```python
from build123d import *

# Parameters (mm, degrees)
SKETCH1_W                   = 76.2
SKETCH1_H                   = 86.36
BOSS_EXTRUDE1_DEPTH         = 12.7
FILLET1_R                   = 3.81
CHAMFER1_SIZE               = 1.27
CUT_EXTRUDE1_DEPTH          = 10.16
SKETCH5_W                   = 16.51
SKETCH5_H                   = 11.43
CUT_EXTRUDE2_DEPTH          = 2.54
CUT_EXTRUDE3_REACH          = 117.87
SKETCH6_W                   = 16.51
SKETCH6_H                   = 7.62
CUT_EXTRUDE4_REACH          = 117.87
SKETCH8_W                   = 8.128
SKETCH8_H                   = 1.27
CUT_EXTRUDE5_REACH          = 117.87
SKETCH9_W                   = 10.16
SKETCH9_H                   = 3.81
CUT_EXTRUDE6_REACH          = 117.87
SKETCH10_W                  = 10.16
SKETCH10_H                  = 7.62
CUT_EXTRUDE7_REACH          = 117.87
SKETCH11_W                  = 26.67
SKETCH11_H                  = 15.24
F_1_4_20_TAPPED_HOLE1_D     = 5.1054
F_1_4_20_TAPPED_HOLE1_DEPTH = 6.35
F_1_4_20_TAPPED_HOLE1_TIP   = 1.533816902


with BuildPart() as part:
    # Sketch1 → Boss-Extrude1 (new body)
    with BuildSketch(Plane(origin=(0, 0, 0), x_dir=(1, 0, 0), z_dir=(0, 1, 0))):
        with Locations((38.1, 43.18)):
            Rectangle(SKETCH1_W, SKETCH1_H)
    extrude(amount=BOSS_EXTRUDE1_DEPTH)

    # Fillet1
    fillet1_edges = [part.edges().sort_by_distance(p)[0] for p in [
        (0, 6.35, -86.36),
        (76.2, 6.35, -86.36),
        (76.2, 6.35, 0),
        (0, 6.35, 0),
    ]]
    fillet(fillet1_edges, radius=FILLET1_R)

    # Chamfer1
    chamfer1_edges = [part.edges().sort_by_distance(p)[0] for p in [
        (0, 12.7, -43.18),
        (38.1, 12.7, -86.36),
        (38.1, 12.7, 0),
        (76.2, 12.7, -43.18),
        (1.115923164, 12.7, -1.115923164),
        (75.084076836, 12.7, -1.115923164),
        (75.084076836, 12.7, -85.244076836),
        (1.115923164, 12.7, -85.244076836),
    ]]
    chamfer(chamfer1_edges, length=CHAMFER1_SIZE)

    # Sketch4 → Cut-Extrude1 (cut)
    with BuildSketch(Plane.XZ):
        Polygon((3.81, -16.51), (16.51, -16.51), (16.51, -3.81), (59.69, -3.81), (59.69, -16.51), (72.39, -16.51), (72.39, -69.85), (59.69, -69.85), (59.69, -82.55), (16.51, -82.55), (16.51, -69.85), (3.81, -69.85), align=None)
    extrude(amount=-CUT_EXTRUDE1_DEPTH, mode=Mode.SUBTRACT)

    # Sketch5 → Cut-Extrude2 (cut)
    with BuildSketch(Plane(origin=(0, 12.7, 0), x_dir=(1, 0, 0), z_dir=(0, 1, 0))):
        with Locations((38.1, 10.795)):
            Rectangle(SKETCH5_W, SKETCH5_H)
    extrude(amount=-CUT_EXTRUDE2_DEPTH, mode=Mode.SUBTRACT)

    # Sketch6 → Cut-Extrude3 (cut, up to next)
    with BuildSketch(Plane.XY, mode=Mode.PRIVATE) as cut_extrude3_sk1:
        with Locations((38.1, 3.81)):
            Rectangle(SKETCH6_W, SKETCH6_H)
    cut_extrude3_tool1 = extrude(cut_extrude3_sk1.sketch, amount=-CUT_EXTRUDE3_REACH, mode=Mode.PRIVATE) & part.part
    add(cut_extrude3_tool1.solids().sort_by_distance((38.1, 3.81, 0))[0], mode=Mode.SUBTRACT)

    # Sketch8 → Cut-Extrude4 (cut, up to next)
    with BuildSketch(Plane(origin=(0, 0, -86.36), x_dir=(-1, 0, 0), z_dir=(0, 0, -1)), mode=Mode.PRIVATE) as cut_extrude4_sk1:
        with Locations((-38.1, 0.635)):
            Rectangle(SKETCH8_W, SKETCH8_H)
    cut_extrude4_tool1 = extrude(cut_extrude4_sk1.sketch, amount=-CUT_EXTRUDE4_REACH, mode=Mode.PRIVATE) & part.part
    add(cut_extrude4_tool1.solids().sort_by_distance((38.1, 0.635, -86.36))[0], mode=Mode.SUBTRACT)

    # Sketch9 → Cut-Extrude5 (cut, up to next)
    with BuildSketch(Plane(origin=(0, 0, -86.36), x_dir=(-1, 0, 0), z_dir=(0, 0, -1)), mode=Mode.PRIVATE) as cut_extrude5_sk1:
        with Locations((-53.34, 1.905)):
            Rectangle(SKETCH9_W, SKETCH9_H)
    cut_extrude5_tool1 = extrude(cut_extrude5_sk1.sketch, amount=-CUT_EXTRUDE5_REACH, mode=Mode.PRIVATE) & part.part
    add(cut_extrude5_tool1.solids().sort_by_distance((53.34, 1.905, -86.36))[0], mode=Mode.SUBTRACT)

    # Sketch10 → Cut-Extrude6 (cut, up to next)
    with BuildSketch(Plane(origin=(0, 12.7, 0), x_dir=(1, 0, 0), z_dir=(0, 1, 0)), mode=Mode.PRIVATE) as cut_extrude6_sk1:
        with Locations((53.34, 77.47)):
            Rectangle(SKETCH10_W, SKETCH10_H)
    cut_extrude6_tool1 = extrude(cut_extrude6_sk1.sketch, amount=-CUT_EXTRUDE6_REACH, mode=Mode.PRIVATE) & part.part
    add(cut_extrude6_tool1.solids().sort_by_distance((53.34, 12.7, -77.47))[0], mode=Mode.SUBTRACT)

    # Sketch11 → Cut-Extrude7 (cut, up to next)
    with BuildSketch(Plane(origin=(0, 12.7, 0), x_dir=(1, 0, 0), z_dir=(0, 1, 0)), mode=Mode.PRIVATE) as cut_extrude7_sk1:
        with Locations((55.88, 44.196)):
            Rectangle(SKETCH11_W, SKETCH11_H)
    cut_extrude7_tool1 = extrude(cut_extrude7_sk1.sketch, amount=-CUT_EXTRUDE7_REACH, mode=Mode.PRIVATE) & part.part
    add(cut_extrude7_tool1.solids().sort_by_distance((55.88, 12.7, -44.196))[0], mode=Mode.SUBTRACT)

    # 1/4-20 Tapped Hole1
    with Locations(Plane(origin=(10.16, 0, -10.16), x_dir=(0, 0, -1), z_dir=(0, -1, 0))):
        with Locations((0, 0), (66.04, 0), (66.04, 55.88), (0, 55.88)):
            Hole(F_1_4_20_TAPPED_HOLE1_D / 2, depth=F_1_4_20_TAPPED_HOLE1_DEPTH)
            with Locations((0, 0, -(F_1_4_20_TAPPED_HOLE1_DEPTH + F_1_4_20_TAPPED_HOLE1_TIP / 2))):  # 118° drill point
                Cone(0, F_1_4_20_TAPPED_HOLE1_D / 2, F_1_4_20_TAPPED_HOLE1_TIP, mode=Mode.SUBTRACT)


solid = part.part
```
Input: part model. Units: mm. Frame: model coordinates. A direction names the side the tool comes from. Give positions to 0.01 mm unless a question says otherwise; leave off trailing zeros. Write each loop counter-clockwise with the first axis right and the second up, starting at its lowest first coordinate (ties: lowest second). Pieces come first, ordered by that corner, then holes. Notation, with made-up numbers: (58.5, 2) - (63.5, 2) arc R21 ccw to (63.5, 9) - close; hole circle Ø10 at (-15, 10). An arc over 180 degrees is marked (long way). Write item = value, one per line. Start each with the question number.
1) Cut plane B-B (x = 40.5). Return loops of the section in (y, z), and give its area (3 significant figures).
2) Cut plane C-C (z = -72.5). Return loops of the section in (x, y), and give its area (3 significant figures).
3) Material intervals for L1, parallel to X at y = 3.25, z = -10.16; L2, parallel to Z at x = 10.16, y = 5; L3, parallel to Z at x = 7, y = 7, sorted ascending. Write a range as [from, to].
4) Pin query (flat end, axial travel): pin 1 (1.1 mm diameter, centred on y = 5, z = -1.5, fed in from -X); pin 2 (5 mm diameter, centred on x = 24.5, z = -68.5, fed in from -Y); pin 3 (4 mm diameter, centred on x = 36.5, y = 3.5, fed in from +Z). Return the tip coordinate at first contact, or that it passes through.
5) Draft query along X for faces 4 (the face through (48.26, 2, -84)), 5 (the face through (38, 6, -86.36)), 6 (the face through (75.054, 5.795, -1.086)), 7 (the face through (38, 11, -5.08)). Return one class per face: pulls with the +X half, pulls with the -X half, needs draft (parallel to the pull), parting line crosses it, or undercut.
6) Cut plane D-D (z = -61). Return loops of the section in (x, y).
7) Reachability of faces 1 (the face through (7.668, 3.219, -10.713)), 2 (the face through (56, 11, -36.576)), 3 (the face through (38, 7.62, -2)) from +Z, -Z, +X, -X, +Y, -Y: full face, straight path, thin tool, end or side. Return the list, or none.
8) Cut plane A-A (z = -39). Return loops of the section in (x, y) (3 decimals), and give its area (3 significant figures).
Answers follow:
q1.outline = (1.27, -86.36) - (11.43, -86.36) - (12.7, -85.09) - (12.7, -16.51) - (10.16, -16.51) - (10.16, -82.55) - (1.27, -82.55) - close; (7.62, -3.81) - (10.16, -3.81) - (10.16, -5.08) - (12.7, -5.08) - (12.7, -1.27) - (11.43, 0) - (7.62, 0) - close
q1.area = 232 mm^2
q2.outline = (0, 0) - (16.51, 0) - (16.51, 10.16) - (59.69, 10.16) - (59.69, 0) - (76.2, 0) - (76.2, 11.43) - (74.93, 12.7) - (1.27, 12.7) - (0, 11.43) - close
q2.area = 527 mm^2
q3.L1 = [0, 7.61], [12.71, 16.51], [59.69, 63.49], [68.59, 76.2]
q3.L2 = [-86.36, -78.75], [-73.65, -69.85], [-16.51, -12.71], [-7.61, 0]
q3.L3 = [-86.36, -69.85], [-16.51, 0]
q4.pin_1 = 0.43
q4.pin_2 = 10.16
q4.pin_3 = -82.55
q5.face_4 = undercut
q5.face_5 = needs draft
q5.face_6 = pulls with the +X half
q5.face_7 = undercut
q6.outline = (0, 0) - (3.81, 0) - (3.81, 10.16) - (72.39, 10.16) - (72.39, 0) - (76.2, 0) - (76.2, 11.43) - (74.93, 12.7) - (1.27, 12.7) - (0, 11.43) - close
q7.face_1 = -Y
q7.face_2 = +Y, -Y
q7.face_3 = +Z, -Y
q8.outline = (0, 0) - (3.81, 0) - (3.81, 10.16) - (42.545, 10.16) - (42.545, 12.7) - (1.27, 12.7) - (0, 11.43) - close; (69.215, 10.16) - (72.39, 10.16) - (72.39, 0) - (76.2, 0) - (76.2, 11.43) - (74.93, 12.7) - (69.215, 12.7) - close
q8.area = 202 mm^2
